Autodesk Inventor part; units mm, degrees
ref_plane "YZ Plane" through (0, 0, 0) normal (1, 0, 0) x (0, 1, 0)
ref_plane "XZ Plane" through (0, 0, 0) normal (0, 1, 0) x (-1, 0, 0)
ref_plane "XY Plane" through (0, 0, 0) normal (0, 0, 1) x (1, 0, 0)
sketch "Sketch1" plane through (0, 0, 0) normal (0, 0, 1) x (1, 0, 0)
  line L0 (4.5611, 7.9) -> (9.1221, 0)
  line L1 (9.1221, 0) -> (4.5611, -7.9)
  line L2 (4.5611, -7.9) -> (-4.5611, -7.9)
  line L3 (-4.5611, -7.9) -> (-9.1221, 0)
  line L4 (-9.1221, 0) -> (-4.5611, 7.9)
  line L5 (-4.5611, 7.9) -> (4.5611, 7.9)
  circle A0 centre (0, 2) radius 1
  circle A1 centre (0, 2) radius 3
  line L6 (4.3301, 7.5) -> (8.6603, 0)
  line L7 (8.6603, 0) -> (4.3301, -7.5)
  line L8 (4.3301, -7.5) -> (-4.3301, -7.5)
  line L9 (-4.3301, -7.5) -> (-8.6603, 0)
  line L10 (-8.6603, 0) -> (-4.3301, 7.5)
  line L11 (-4.3301, 7.5) -> (4.3301, 7.5)
  line L12 (4.1, 3.75) -> (4.1, 0.25)
  line L13 (4.1, 0.25) -> (4.9, 0.25)
  line L14 (4.9, 0.25) -> (4.9, 3.75)
  line L15 (4.9, 3.75) -> (4.1, 3.75)
  line L16 (0.38, -3.1) -> (3.38, -3.1)
  line L17 (3.38, -3.1) -> (3.38, -3.7)
  line L18 (3.38, -3.7) -> (0.38, -3.7)
  line L19 (0.38, -3.7) -> (0.38, -3.1)
  line L20 (-3.02, -0.95) -> (-0.02, -0.95)
  line L21 (-0.02, -0.95) -> (-0.02, -1.55)
  line L22 (-0.02, -1.55) -> (-3.02, -1.55)
  line L23 (-3.02, -1.55) -> (-3.02, -0.95)
  line L24 (-4.5, 4.5) -> (4.5, 4.5)
  line L25 (4.5, 4.5) -> (4.5, -4.5)
  line L26 (4.5, -4.5) -> (-4.5, -4.5)
  line L27 (-4.5, -4.5) -> (-4.5, 4.5)
  circle A2 centre (0, 0) radius 6.5
  line L28 (-5.8, -5.8) -> (5.8, -5.8)
  line L29 (5.8, -5.8) -> (5.8, 5.8)
  line L30 (5.8, 5.8) -> (-5.8, 5.8)
  line L31 (-5.8, 5.8) -> (-5.8, -5.8)
  point P0 (-2.9343, -5.8)
  point P1 (2.9343, -5.8)
  point P2 (2.9343, 5.8)
  point P3 (-2.9343, 5.8)
  point P4 (5.8, -5.7541)
  point P5 (5.8, 5.7541)
  point P6 (5.7735, 5.8)
  point P7 (-5.7735, 5.8)
  point P8 (-5.8, 5.7541)
  point P9 (-5.8, -5.7541)
  point P10 (-5.7735, -5.8)
  point P11 (5.7735, -5.8)
extrude "Extrusion4" add sketch "Sketch1" against normal blind 9 contours A2 L29 L28 L31 L30 | A2 L29 | L31 A2 | A1 L24 L25 L15 L12 L13 L26 L27 L20 L23 L22 L21 | L21 L22 L23 L20 A1 | L25 L13 L12 L15 | L15 L14 L13 L25 | L16 L17 L18 L19
extrude "Extrusion5" add sketch "Sketch1" against normal blind 2 from surface at -9 contours L0 L30 L6 L11 L10 L4 L5 | L0 L29 L6 L30 | L0 L1 L29 L7 L6 | L30 A2 L10 L11 L6 | L6 L29 A2 L30 | L30 L10 L31 L4 | L6 L7 L29 A2 | L30 A2 | A2 L29 L28 L31 L30 | L31 L10 L9 L3 L4 | L30 A2 L31 L10 | L1 L28 L7 L29 | A2 L29 | L31 A2 L9 L10 | L1 L2 L3 L28 L9 L8 L7 | L7 L28 A2 L29 | L31 A2 | L31 L9 L28 L3 | L7 L8 L9 L28 A2 | A2 L28 | A2 L28 L9 L31 | A0 | A1 L21 L20 L24 | A1 L24 L25 L15 L12 L13 L26 L27 L20 L23 L22 L21 | L24 A1 | L21 L22 L23 L20 A1 | A1 L20 L21 | L25 L13 L12 L15 | L15 L14 L13 L25 | L16 L17 L18 L19
extrude "Extrusion6" add sketch "Sketch1" against normal blind 2 from surface at -11 contours A0 | A1 L21 L20 L24 | A1 L24 L25 L15 L12 L13 L26 L27 L20 L23 L22 L21 | L21 L22 L23 L20 A1 | A1 L20 L21 | L25 L13 L12 L15 | L16 L17 L18 L19
extrude "Extrusion7" add sketch "Sketch1" against normal blind 4.9 from surface at -13 contours L21 L22 L23 L20 A1 | A1 L20 L21 | L16 L17 L18 L19
extrude "Extrusion8" add sketch "Sketch1" against normal blind 6 from surface at -11 contours L25 L13 L12 L15 | L15 L14 L13 L25
extrude "Extrusion9" add sketch "Sketch1" along normal blind 6.3 from surface at -9 contours L30 A2 L10 L11 L6 | L6 L29 A2 L30 | L6 L7 L29 A2 | L30 A2 L31 L10 | L31 A2 L9 L10 | L7 L28 A2 L29 | L7 L8 L9 L28 A2 | A2 L28 L9 L31
extrude "Extrusion10" cut sketch "Sketch1" along normal blind 4 from surface at -9 contours L30 A2 L10 L11 L6 | L6 L29 A2 L30 | L6 L7 L29 A2 | L30 A2 L31 L10 | L31 A2 L9 L10 | L7 L28 A2 L29 | L7 L8 L9 L28 A2 | A2 L28 L9 L31
extrude "Extrusion11" add sketch "Sketch1" along normal blind 8 from surface at -9 contours A0
properties part number "Jack"
Part model, mm, in its own coordinate system. A direction names the side the tool comes from. Give positions to 0.01 mm unless a question says otherwise; leave off trailing zeros. Order: outer loops, then holes, each group sorted by start corner. A loop starts at its lowest first (then second) coordinate and runs counter-clockwise, first axis right, second up. Notation, with made-up numbers: M 70.5,53.25 L 89.5,53.25 A19 cw 89.5,90.25 Z; hole C 47,-12.5 d4. An arc over 180 degrees is marked long. Use a Markdown table: item, result. Add a question column.
(1) Saw through at A-A, the plane z = -3.5. Give the cut face in (x, y).
(2) 3-axis set-ups, long thin cutter, end or side, ignore diameter. For faces 5 (the face through (0, 4.5, -12)), 6 (the face through (0, -4.5, -12)), 7 (the face through (6.5, 0.1, -7)): which of +Z, -Z, +X, -X, +Y, -Y reach the whole face in a straight line?
(3) Saw through at C-C, the plane y = -7. Give the cut face in (x, z), and give its area (3 significant figures).
(4) Probe line 1 along Y through (x, z) = (0, -2); line 2 along Y through (x, z) = (4.5, -13.25); line 3 along X through (y, z) = (0.75, -3.5). List the from-to ranges inside material, lowest first. Write a range as [from, to].
(5) Mould opens along X. For faces 1 (the face through (4.1, 2, -15)), 2 (the face through (6.81, 4.005, -9.986)), 3 (the face through (0, -5.8, -4)), 4 (the face through (4.5, 0.25, -14.6)) say: +X half, -X half, draft (parallel to the pull), parting line (faces both ways), or undercut.
(6) Saw through at D-D, the plane z = -12.5. Give the cut face in (x, y).
(7) Drop flat-ended pins along their axis: P1, Ø0.9, axis at x = 2.5, z = -15.5, coming from the -Y side; P2, Ø4, axis at x = -0.5, z = -6, coming from the -Y side; P3, Ø0.7, axis at y = -1.5, z = -16.5, coming from the -X side. Give the stop position or say it passes through.
(8) Saw through at B-B, the plane x = -7. Give the cut face in (y, z).
Answer key:
| question | item | result |
|---|---|---|
| 1 | outline | M -8.66,0 L -4.33,-7.5 L 4.33,-7.5 L 8.66,0 L 4.33,7.5 L -4.33,7.5 Z; C 0,2 d2; hole C 0,2 d6; hole M -2.93,-5.8 A6.5 ccw 2.93,-5.8 Z; hole M -2.93,5.8 L 2.93,5.8 A6.5 ccw Z |
| 2 | face 5 | -Z, +X, -X, +Y |
| 2 | face 6 | -Z, +X, -X, -Y |
| 2 | face 7 | +X |
| 3 | outline | M -5.08,-11 L 5.08,-11 L 5.08,-9 L -5.08,-9 Z; M -4.62,-5 L 4.62,-5 L 4.62,-2.7 L -4.62,-2.7 Z |
| 3 | area | 41.6 mm^2 |
| 4 | line 1 | [-5.8, -1], [1, 3], [5, 5.8] |
| 4 | line 2 | [0.25, 3.75] |
| 4 | line 3 | [-8.23, -2.73], [2.73, 8.23] |
| 5 | face 1 | -X half |
| 5 | face 2 | +X half |
| 5 | face 3 | undercut |
| 5 | face 4 | draft |
| 6 | outline | M -4.5,-4.5 L 4.5,-4.5 L 4.5,0.25 L 4.9,0.25 L 4.9,3.75 L 4.5,3.75 L 4.5,4.5 L -4.5,4.5 Z |
| 7 | P1 | y = -3.7 |
| 7 | P2 | y = -7.5 |
| 7 | P3 | x = -3.02 |
| 8 | outline | M -3.68,-11 L 3.68,-11 L 3.68,-9 L -3.68,-9 Z; M -2.88,-5 L 2.88,-5 L 2.88,-2.7 L -2.88,-2.7 Z |
